Check sheet for the drawn part. Datum: minimum x, y, z corner. Units: mm. A direction names the side the tool comes from. Round coordinates to 2 decimals unless told otherwise and drop trailing zeros. Write each loop counter-clockwise with the first axis right and the second up, starting at its lowest first coordinate (ties: lowest second). Pieces come first, ordered by that corner, then holes. Notation, with made-up numbers: (80, -33) -> (92, -33) arc R34 ccw to (92, 1) -> close; hole circle Ø6 at (85.25, 84). An arc over 180 degrees is marked (long way). One line per item, written item: value. Start each with the question number.
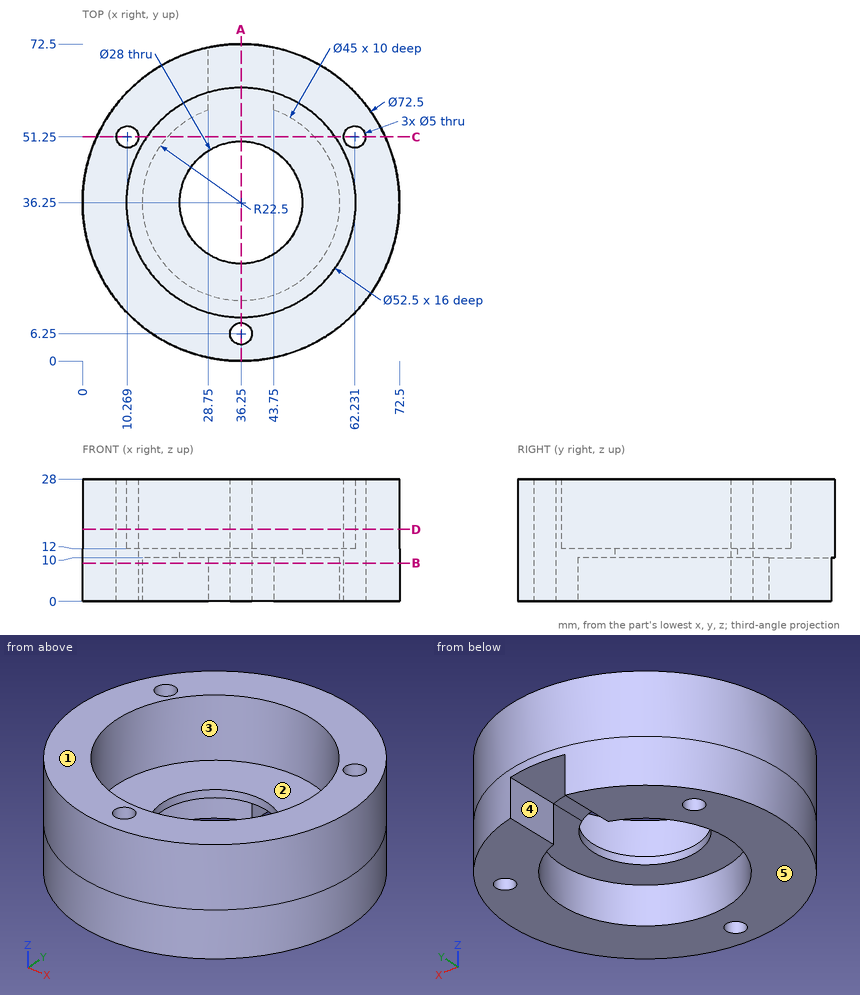
1. Release check for a two-part mould opening along X. For the marked faces 1 and 2 record: +X half, -X half, draft (parallel to the pull), parting line (faces both ways), or undercut.
2. Cross-section at B-B (z = 8.75). Record the cut outline in (x, y).
3. Cross-section at C-C (y = 51.25). Record the cut outline in (x, z).
4. Cross-section at D-D (z = 16.5). Record the cut outline in (x, y).
5. Access from +Z, -Z, +X, -X, +Y, -Y to the whole of each face (thin tool, end or side, straight path). Record for the marked faces 3, 4 and 5.
6. Cross-section at A-A (x = 36.25). Record the cut outline in (y, z).
7. Depth check by flat-ended pin: pin 1 Ø12 at (x, y) = (36.5, 65) entering from -Z; pin 2 Ø4 at (x, z) = (20.5, 20) entering from -Y; pin 3 Ø10 at (x, z) = (62, 22) entering from +Y. Enter the tip coordinate at first touch or a pass-through.
8. Material ranges on probe 1 along Y at (x, z) = (36.25, 13.5); probe 2 along Y at (x, z) = (36.25, 5.75); probe 3 along X at (y, z) = (50, 13) (1 decimal), recorded low to high.
Working result:
1. face 1: draft
1. face 2: undercut
2. outline: (28.75, 57.46) -> (28.75, 71.72) arc R36.25 ccw (long way) to (43.75, 71.72) -> (43.75, 57.46) arc R22.5 cw (long way) to start; hole circle Ø5 at (10.27, 51.25); hole circle Ø5 at (36.25, 6.25); hole circle Ø5 at (62.23, 51.25)
3. outline: (3.25, 0) -> (7.77, 0) -> (7.77, 28) -> (3.25, 28) -> close; (12.77, 0) -> (19.48, 0) -> (19.48, 10) -> (53.02, 10) -> (53.02, 0) -> (59.73, 0) -> (59.73, 28) -> (57.79, 28) -> (57.79, 12) -> (14.71, 12) -> (14.71, 28) -> (12.77, 28) -> close; (64.73, 0) -> (69.25, 0) -> (69.25, 28) -> (64.73, 28) -> close
4. outline: circle Ø72.5 at (36.25, 36.25); hole circle Ø5 at (10.27, 51.25); hole circle Ø52.5 at (36.25, 36.25); hole circle Ø5 at (36.25, 6.25); hole circle Ø5 at (62.23, 51.25)
5. face 3: +Z
5. face 4: -Z, +Y
5. face 5: -Z, +X, -X, +Y, -Y
6. outline: (0, 0) -> (3.75, 0) -> (3.75, 28) -> (0, 28) -> close; (8.75, 0) -> (13.75, 0) -> (13.75, 10) -> (22.25, 10) -> (22.25, 12) -> (10, 12) -> (10, 28) -> (8.75, 28) -> close; (50.25, 10) -> (72.5, 10) -> (72.5, 28) -> (62.5, 28) -> (62.5, 12) -> (50.25, 12) -> close
7. pin 1: stops at z = 10
7. pin 2: stops at y = 2.71
7. pin 3: stops at y = 65.97
8. probe 1: y = 0 to 3.75, 8.75 to 10, 62.5 to 72.5
8. probe 2: y = 0 to 3.75, 8.75 to 13.75
8. probe 3: x = 2.7 to 8.1, 12.4 to 13.9, 58.6 to 60.1, 64.4 to 69.8
